CAD build for the part. Positions are in the model's coordinates, mm. A direction names the side the tool comes from. Round coordinates to 2 decimals unless told otherwise and drop trailing zeros. Write each loop counter-clockwise with the first axis right and the second up, starting at its lowest first coordinate (ties: lowest second). Pieces come first, ordered by that corner, then holes. Notation, with made-up numbers: (50, 3.5) - (90, 3.5) arc R14 cw to (90, 13.5) - close; hole circle Ø5 at (-5, 18). An arc over 180 degrees is marked (long way). Put each result on its own line as item: value. Start each with the question number.
Item 1: Cut at C-C (z = -22). Give the cut face in (x, y).
Item 2: Cut at B-B (x = 26). Give the cut face in (y, z).
Item 3: 3-axis set-ups, long thin cutter, end or side, ignore diameter. For faces 1 (the cylindrical face through (15.01, 214.79, -7.85)), 2 (the cylindrical face through (31.923, 122.535, -28.226)), 3 (the flat face through (12, 192, -30)), 4 (the cylindrical face through (15.01, 22.85, -30.42)): which of +Z, -Z, +X, -X, +Y, -Y reach the whole face in a straight line?
Item 4: Cut at A-A (y = 207). Give the cut face in (x, z).
Item 5: Cut at D-D (x = 39.5). Give the cut face in (y, z), and give its area (3 significant figures).
Item 6: Drill centre lines: line 1 (Z direction, x = 26, y = 14.5); line 2 (Y direction, x = 44.5, z = -31.5); line 3 (Y direction, x = 31.5, z = -3.5). Where is each one in solid material? Low to high. Write a range as from..to.
Item 7: Mould opens along Z. For faces 5 (the flat face through (10, 97, -60)), 6 (the flat face through (32, 200, -3)), 7 (the cylindrical face through (6, 82, -38)) say: released by +Z, released by -Z, zero draft, split by the parting line, or undercut.
Item 8: Pin check, flat tips, straight feed: pin 1 Ø10 at (x, z) = (34, -41.5) entering from +Y; pin 2 Ø8 at (y, z) = (62, -46.5) entering from -X; pin 3 Ø6 at (x, z) = (4, -23.5) entering from +Y; pin 4 Ø2.5 at (y, z) = (148.5, -41) entering from +X. Stop position of each tip, or through.
Autodesk Inventor part; units mm, degrees
ref_plane "YZ Plane" through (0, 0, 0) normal (1, 0, 0) x (0, 1, 0)
ref_plane "XZ Plane" through (0, 0, 0) normal (0, 1, 0) x (-1, 0, 0)
ref_plane "XY Plane" through (0, 0, 0) normal (0, 0, 1) x (1, 0, 0)
sketch "Эскиз1" plane through (0, 0, 0) normal (0, 1, 0) x (-1, 0, 0)
  line L0 (0, 0) -> (-60, 0)
  line L1 (-60, 0) -> (-60, -60)
  line L2 (-60, -60) -> (0, -60)
  line L3 (0, -60) -> (0, 0)
  dimension "d0" = 60
  dimension "d1" = 60
extrude "Выдавливание1" add sketch "Эскиз1" along normal blind 20
sketch "Эскиз2" plane through (0, 20, 0) normal (0, 1, 0) x (1, 0, 0)
  line L0 (0, 0) -> (60, 0)
  line L1 (0, 0) -> (12, 0)
  line L2 (12, 0) -> (12, 60)
  line L3 (60, 60) -> (0, 60)
  line L4 (0, 60) -> (0, 0)
  line L5 (0, 60) -> (0, 0)
  dimension "d4" = 12
extrude "Выдавливание2" add sketch "Эскиз2" along normal blind 260
sketch "Эскиз3" plane through (0, 20, 0) normal (0, 1, 0) x (1, 0, 0)
  point P0 (0, 0)
  point P1 (26, 13)
  point P2 (26, 47)
  point P3 (50.2241, 13)
  point P4 (50.2241, 47)
hole "Отверстие1" at (26, 20, -13) at (26, 20, -47) at (50.2241, 20, -13) at (50.2241, 20, -47) direction (0, -1, 0) diameter 4 depth 40 tip angle 118
sketch "Эскиз4" plane through (12, 20, 0) normal (1, 0, 0) x (0, 0, -1)
  point P0 (0, -20)
  point P1 (30, 88)
  dimension "d14" = 0
extrude "Выдавливание3" [suppressed]
sketch "Эскиз5" plane through (12, 20, 0) normal (1, 0, 0) x (0, 0, -1)
  point P0 (0, -20)
sketch "Эскиз6" plane through (0, 0, 0) normal (0, 0, 1) x (1, 0, 0)
  line L0 (0, 0) -> (0, 280)
  line L1 (12, 20) -> (12, 280)
sketch "Эскиз7" plane through (60, 0, -60) normal (0, 0, -1) x (-1, 0, 0)
  point P0 (60, 0)
sketch "Эскиз8" plane through (12, 20, 0) normal (1, 0, 0) x (0, 0, -1)
  circle A0 centre (30, 80) radius 11.5
  point P0 (0, -20)
  point P1 (0, 80)
  dimension "d17" = 23
extrude "Выдавливание4" cut sketch "Эскиз8" against normal blind 100
sketch "Эскиз9" plane through (0, 0, -60) normal (-1, 0, 0) x (0, 0, 1)
  circle A0 centre (29.731, 99.8395) radius 12.5286
  point P0 (60, 0)
  point P1 (0, 80)
extrude "Выдавливание5" add sketch "Эскиз9" against normal blind 12
sketch "Эскиз10" plane through (0, 0, -60) normal (-1, 0, 0) x (0, 0, 1)
  line L0 (0, 0) -> (0, 280)
  circle A0 centre (30, 60) radius 11
  circle A1 centre (22, 80) radius 2
  circle A2 centre (38, 80) radius 2
  point P0 (60, 0)
  point P1 (0, 60)
  point P2 (0, 80)
  point P3 (30, 80)
  dimension "d22" = 22
  dimension "d23" = 4
  dimension "d24" = 4
extrude "Выдавливание6" cut sketch "Эскиз10" against normal blind 12
sketch "Эскиз11" plane through (0, 0, 0) normal (0, -1, 0) x (1, 0, 0)
  point P0 (0, 0)
fillet "Сопряжение1" radius 10 1 edges at (12, 20, -30)
sketch "Эскиз12" plane through (0, 0, -60) normal (-1, 0, 0) x (0, 0, 1)
  line L0 (0, 120) -> (60, 120)
  line L1 (60, 120) -> (60, 125)
  line L2 (60, 125) -> (0, 125)
  line L3 (0, 125) -> (0, 120)
  point P0 (60, 0)
  dimension "d28" = 60
  dimension "d29" = 5
extrude "Выдавливание7" add sketch "Эскиз12" against normal blind 50
fillet "Сопряжение2" radius 5 1 edges at (12, 125, -30)
sketch "Эскиз13" plane through (50, 125, 0) normal (0, 1, 0) x (1, 0, 0)
  circle A0 centre (-19, 30) radius 2
  point P0 (-50, 0)
  dimension "d33" = 4
extrude "Выдавливание8" cut sketch "Эскиз13" against normal blind 50
sketch "Эскиз14" plane through (0, 0, -60) normal (-1, 0, 0) x (0, 0, 1)
  line L0 (0, 0) -> (0, 280)
  line L1 (0, 145) -> (60, 145)
  line L2 (60, 145) -> (60, 150)
  line L3 (60, 150) -> (0, 150)
  line L4 (0, 150) -> (0, 145)
  point P0 (60, 0)
  dimension "d36" = 60
  dimension "d37" = 5
extrude "Выдавливание9" add sketch "Эскиз14" against normal blind 50
fillet "Сопряжение3" radius 5 1 edges at (12, 150, -30)
sketch "Эскиз15" plane through (12, 145, -60) normal (0, -1, 0) x (1, 0, 0)
  circle A0 centre (19, 30) radius 2
  circle A1 centre (19, 30) radius 2
  circle A2 centre (19, 30) radius 2
  point P0 (-12, 60)
  point P1 (3.4297, 11.4015)
  dimension "d41" = 4
extrude "Выдавливание10" cut sketch "Эскиз15" against normal blind 50
sketch "Эскиз16" plane through (0, 0, -60) normal (-1, 0, 0) x (0, 0, 1)
  line L0 (0, 0) -> (0, 280)
  circle A0 centre (30, 215) radius 0.5
  point P0 (60, 0)
  point P1 (0, 215)
  point P2 (0, 215)
  dimension "d44" = 1
extrude "Выдавливание11" cut sketch "Эскиз16" against normal blind 100
sketch "Эскиз17" plane through (12, 280, 0) normal (1, 0, 0) x (0, 0, -1)
  point P0 (0, -280)
sketch "Эскиз18" plane through (12, 280, 0) normal (1, 0, 0) x (0, 0, -1)
  line L0 (0, -125) -> (0, 0)
  line L1 (60, -280) -> (60, 0)
  line L2 (0, -80) -> (0, -50)
  line L3 (0, -50) -> (5, -50)
  line L4 (5, -50) -> (5, -80)
  line L5 (5, -80) -> (0, -80)
  line L6 (0, -80) -> (0, -50)
  point P0 (0, -280)
  point P1 (30, -80)
  point P2 (30, -50)
  dimension "d47" = 5
extrude "Выдавливание12" add sketch "Эскиз18" along normal blind 44.5
sketch "Эскиз19" plane through (0, 0, 0) normal (0, 0, 1) x (1, 0, 0)
  circle A0 centre (52.5, 223) radius 2
  circle A1 centre (52.5, 207) radius 2
  point P0 (0, 0)
  point P1 (52.5, 215)
  dimension "d50" = 4
  dimension "d51" = 4
extrude "Выдавливание13" cut sketch "Эскиз19" against normal blind 45
fillet "Сопряжение4" radius 10 1 edges at (12, 215, -5)
sketch "Эскиз20" plane through (12, 280, 0) normal (1, 0, 0) x (0, 0, -1)
  line L0 (0, -280) -> (0, 0)
  line L1 (0, -50.033) -> (60, -50.033)
  line L2 (60, -280) -> (60, 0)
  line L3 (60, -50.033) -> (60, 0)
  line L4 (60, 0) -> (0, 0)
  line L5 (0, 0) -> (0, -50.033)
extrude "Выдавливание14" cut sketch "Эскиз20" against normal blind 100
properties part number "Подпора"
Output values:
1. outline: (0, 0) - (60, 0) - (60, 20) - (22, 20) arc R10 cw to (12, 30) - (12, 52.45) - (0, 52.45) - close; (0, 67.55) - (12, 67.55) - (12, 78) - (0, 78) - close; (0, 82) - (12, 82) - (12, 120) - (50, 120) - (50, 125) - (17, 125) arc R5 cw to (12, 130) - (12, 145) - (50, 145) - (50, 150) - (17, 150) arc R5 cw to (12, 155) - (12, 229.97) - (0, 229.97) - close
2. outline: (0, -60) - (20, -60) - (20, -49) - (0, -49) - close; (0, -45) - (20, -45) - (20, -15) - (0, -15) - close; (0, -11) - (20, -11) - (20, 0) - (0, 0) - close; (120, -60) - (125, -60) - (125, 0) - (120, 0) - close; (145, -60) - (150, -60) - (150, 0) - (145, 0) - close; (200, -5) - (230, -5) - (230, 0) - (200, 0) - close
3. face 1: -Z, +X, +Y
3. face 2: +Y
3. face 3: -Z, +X
3. face 4: +Z, -Z, +X
4. outline: (0, -60) - (12, -60) - (12, -15) arc R10 cw to (22, -5) - (50.5, -5) - (50.5, 0) - (0, 0) - close; (54.5, -5) - (56.5, -5) - (56.5, 0) - (54.5, 0) - close
5. outline: (0, -60) - (20, -60) - (20, 0) - (0, 0) - close; (120, -60) - (125, -60) - (125, 0) - (120, 0) - close; (145, -60) - (150, -60) - (150, 0) - (145, 0) - close; (200, -5) - (230, -5) - (230, 0) - (200, 0) - close
5. area: 1,950 mm2
6. line 1: -60..-49, -45..-15, -11..0
6. line 2: 0..20, 120..125, 145..150
6. line 3: 0..20, 120..125, 145..150, 200..230
7. face 5: released by -Z
7. face 6: zero draft
7. face 7: undercut
8. pin 1: y = 150
8. pin 2: x = 0
8. pin 3: y = 229.97
8. pin 4: x = 50
